Verification items for the finished model (mm, model axes). A direction names the side the tool comes from. Give positions to 0.01 mm unless a question says otherwise; leave off trailing zeros. Loops run counter-clockwise (first coordinate to the right, second up) from the corner with the lowest first, then second, coordinate; pieces in that order, holes last. Notation, with made-up numbers: M 74,50.5 L 87,50.5 A18 cw 87,74.5 Z; hole C -26.5,46 d7. An arc over 180 degrees is marked long. Use a Markdown table: item, result.
from build123d import *

# Parameters (mm, degrees)
SKETCH1_R           = 50
BOSS_EXTRUDE1_DEPTH = 20
SKETCH2_R           = 50
BOSS_EXTRUDE2_DEPTH = 5
SKETCH3_R           = 2.1
CUT_EXTRUDE1_DEPTH  = 5
SKETCH4_R           = 3.1
CUT_EXTRUDE2_DEPTH  = 76
CUT_EXTRUDE3_DEPTH  = 6
FILLET1_R           = 0.5
CUT_EXTRUDE4_DEPTH  = 76
FILLET2_R           = 10


with BuildPart() as part:
    # Sketch1 → Boss-Extrude1 (new body)
    with BuildSketch(Plane.XY):
        Circle(SKETCH1_R)
        with BuildLine():
            Line((-8.972179222, 12.02081528), (8.972179222, 12.02081528))
            ThreePointArc((8.972179222, 12.02081528), (10.606601718, 10.606601718), (12.02081528, 8.972179222))
            Line((12.02081528, 8.972179222), (12.02081528, -8.972179222))
            ThreePointArc((12.02081528, -8.972179222), (10.606601708, -10.606601708), (8.972179222, -12.02081528))
            Line((8.972179222, -12.02081528), (-8.972179222, -12.02081528))
            ThreePointArc((-8.972179222, -12.02081528), (-10.606601718, -10.606601718), (-12.02081528, -8.972179222))
            Line((-12.02081528, -8.972179222), (-12.02081528, 8.972179222))
            ThreePointArc((-12.02081528, 8.972179222), (-10.606601718, 10.606601718), (-8.972179222, 12.02081528))
        make_face(mode=Mode.SUBTRACT)
    extrude(amount=BOSS_EXTRUDE1_DEPTH)

    # Sketch2 → Boss-Extrude2 (add)
    with BuildSketch(Plane.XY.offset(20)):
        Circle(SKETCH2_R)
    extrude(amount=BOSS_EXTRUDE2_DEPTH)

    # Sketch3 → Cut-Extrude1 (cut)
    with BuildSketch(Plane(origin=(0, 0, 20), x_dir=(-1, 0, 0), z_dir=(0, 0, -1))):
        with Locations((-5.303300859, 5.303300859)):
            Circle(SKETCH3_R)
        with Locations((5.303300859, -5.303300859)):
            Circle(SKETCH3_R)
    extrude(amount=-CUT_EXTRUDE1_DEPTH, mode=Mode.SUBTRACT)

    # Sketch4 → Cut-Extrude2 (cut, through all)
    with BuildSketch(Plane(origin=(0, 0, 0), x_dir=(-1, 0, 0), z_dir=(0, 0, -1))):
        with Locations((0, 30)):
            Circle(SKETCH4_R)
        with Locations((0, -30)):
            Circle(SKETCH4_R)
    extrude(amount=-CUT_EXTRUDE2_DEPTH, mode=Mode.SUBTRACT)

    # Sketch5 → Cut-Extrude3 (cut)
    with BuildSketch(Plane(origin=(0, 0, 0), x_dir=(-1, 0, 0), z_dir=(0, 0, -1))):
        Polygon((5.831237719, 30), (2.915618859, 35.05), (-2.915618859, 35.05), (-5.831237719, 30), (-2.915618859, 24.95), (2.915618859, 24.95), align=None)
        Polygon((5.831237719, -30), (2.915618859, -24.95), (-2.915618859, -24.95), (-5.831237719, -30), (-2.915618859, -35.05), (2.915618859, -35.05), align=None)
    extrude(amount=-CUT_EXTRUDE3_DEPTH, mode=Mode.SUBTRACT)

    # Fillet1
    fillet1_edges = [part.edges().sort_by_distance(p)[0] for p in [
        (-4.373428289, 27.475, 0),
        (-4.373428289, 32.525, 0),
        (0, 35.05, 0),
        (4.373428289, 32.525, 0),
        (4.373428289, 27.475, 0),
        (0, 24.95, 0),
        (-4.373428289, -32.525, 0),
        (-4.373428289, -27.475, 0),
        (0, -24.95, 0),
        (4.373428289, -27.475, 0),
        (4.373428289, -32.525, 0),
        (0, -35.05, 0),
    ]]
    fillet(fillet1_edges, radius=FILLET1_R)

    # Sketch6 → Cut-Extrude4 (cut, through all)
    with BuildSketch(Plane(origin=(0, 0, 0), x_dir=(-1, 0, 0), z_dir=(0, 0, -1))):
        with BuildLine():
            Line((-35, 0), (-35, 35.707142143))
            ThreePointArc((-35, 35.707142143), (-50, 0), (-35, -35.707142143))
            Line((-35, -35.707142143), (-35, 0))
        make_face()
    cut_extrude4 = extrude(amount=-CUT_EXTRUDE4_DEPTH, mode=Mode.SUBTRACT)

    # Mirror1: Cut-Extrude4 across plane
    add(cut_extrude4.mirror(Plane(origin=(0, 0, 0), x_dir=(0, 0, 1), z_dir=(1, 0, 0))), mode=Mode.SUBTRACT)

    # Fillet2
    fillet2_edges = [part.edges().sort_by_distance(p)[0] for p in [
        (35, -35.707142143, 12.5),
        (35, 35.707142143, 12.5),
        (-35, -35.707142143, 12.5),
        (-35, 35.707142143, 12.5),
    ]]
    fillet(fillet2_edges, radius=FILLET2_R)


solid = part.part
(1) Cross-section at B-B on x = 0. Record the cut outline in (y, z).
Results below:
| item | result |
|---|---|
| outline | M -50,0 L -35.55,0 A0.5 ccw -35.05,0.5 L -35.05,6 L -33.1,6 L -33.1,25 L -50,25 Z; M -26.9,6 L -24.95,6 L -24.95,0.5 A0.5 ccw -24.45,0 L -12.02,0 L -12.02,20 L 12.02,20 L 12.02,0 L 24.45,0 A0.5 ccw 24.95,0.5 L 24.95,6 L 26.9,6 L 26.9,25 L -26.9,25 Z; M 33.1,6 L 35.05,6 L 35.05,0.5 A0.5 ccw 35.55,0 L 50,0 L 50,25 L 33.1,25 Z |
(2) Gauge pin test, flat ends, axial feed: P1, Ø11, axis at x = 2.5, y = -30, coming from the -Z side; P2, Ø3, axis at x = -2.5, y = 31, coming from the -Z side; P3, Ø3.5, axis at x = -5.3, y = -5.3, coming from the -Z side; P4, Ø12, axis at x = -3.5, y = 2.5, coming from the -Z side. Record the tip position at first contact, or that the pin passes through.
Results below:
| item | result |
|---|---|
| P1 | z = 0 |
| P2 | z = 6 |
| P3 | through |
| P4 | z = 20 |
(3) Material ranges on line 1 (Y direction, x = 1, z = 14.75); line 2 (X direction, y = -2, z = 16.25); line 3 (Z direction, x = -6, y = 11.5), recorded low to high.
Results below:
| item | result |
|---|---|
| line 1 | -49.99 to -32.93, -27.07 to -12.02, 12.02 to 27.07, 32.93 to 49.99 |
| line 2 | -35 to -12.02, 12.02 to 35 |
| line 3 | 20 to 25 |
(4) Draft check along X on faces 1 (the cylindrical face through (-4.481, 32.639, 0.143)), 2 (the flat face through (-35, 0, 12)), 3 (the cylindrical face through (33.987, 35.612, 12.675)), 4 (the flat face through (0, -12.021, 10)). Enter one of: +X half, -X half, draft (parallel to the pull), parting line (faces both ways), or undercut.
Results below:
| item | result |
|---|---|
| face 1 | undercut |
| face 2 | -X half |
| face 3 | +X half |
| face 4 | undercut |
(5) Set-up check for faces 5 (the flat face through (0, 12.021, 10)), 6 (the cylindrical face through (0, -50, 12)): record each of +Z, -Z, +X, -X, +Y, -Y from which the full face is reachable in a straight line by a thin tool's end or side.
Results below:
| item | result |
|---|---|
| face 5 | -Z |
| face 6 | +Z, -Z, -Y |
(6) Cross-section at D-D on z = 22.5. Record the cut outline in (x, y).
Results below:
| item | result |
|---|---|
| outline | M -35,-31.22 A10 ccw -31.25,-39.03 A50 ccw 31.25,-39.03 A10 ccw 35,-31.22 L 35,31.22 A10 ccw 31.25,39.03 A50 ccw -31.25,39.03 A10 ccw -35,31.22 Z; hole C -5.3,-5.3 d4.2; hole C 0,-30 d6.2; hole C 0,30 d6.2; hole C 5.3,5.3 d4.2 |
(7) Cross-section at A-A on z = 14. Record the cut outline in (x, y).
Results below:
| item | result |
|---|---|
| outline | M -35,-31.22 A10 ccw -31.25,-39.03 A50 ccw 31.25,-39.03 A10 ccw 35,-31.22 L 35,31.22 A10 ccw 31.25,39.03 A50 ccw -31.25,39.03 A10 ccw -35,31.22 Z; hole M -12.02,-8.97 A15 ccw -8.97,-12.02 L 8.97,-12.02 A15 ccw 12.02,-8.97 L 12.02,8.97 A15 ccw 8.97,12.02 L -8.97,12.02 A15 ccw -12.02,8.97 Z; hole C 0,-30 d6.2; hole C 0,30 d6.2 |
(8) Cross-section at C-C on z = 5. Record the cut outline in (x, y), then the cut area to 3 significant figures.
Results below:
| item | result |
|---|---|
| outline | M -35,-31.22 A10 ccw -31.25,-39.03 A50 ccw 31.25,-39.03 A10 ccw 35,-31.22 L 35,31.22 A10 ccw 31.25,39.03 A50 ccw -31.25,39.03 A10 ccw -35,31.22 Z; hole M -12.02,-8.97 A15 ccw -8.97,-12.02 L 8.97,-12.02 A15 ccw 12.02,-8.97 L 12.02,8.97 A15 ccw 8.97,12.02 L -8.97,12.02 A15 ccw -12.02,8.97 Z; hole M -5.83,-30 L -2.92,-35.05 L 2.92,-35.05 L 5.83,-30 L 2.92,-24.95 L -2.92,-24.95 Z; hole M -5.83,30 L -2.92,24.95 L 2.92,24.95 L 5.83,30 L 2.92,35.05 L -2.92,35.05 Z |
| area | 5,630 mm^2 |
